Work out the finished part from the listing and answer in its coordinate system (mm). Round coordinates to 2 decimals unless told otherwise and drop trailing zeros. Order: outer loops, then holes, each group sorted by start corner. A loop starts at its lowest first (then second) coordinate and runs counter-clockwise, first axis right, second up. Notation, with made-up numbers: (21.25, 29.5) - (30.25, 29.5) arc R9 ccw to (30.25, 36.5) - close; hole circle Ø4 at (-22, -26.75). An arc over 180 degrees is marked (long way). Use one line per item in the form item = value. Start each with the question number.
Q1. The part is cut by section A-A on x = 328. Determine the outline of the cut face in (y, z), plus the area to 3 significant figures.
Q2. Find the intervals of material crossed by line 1 (X direction, y = 2.5, z = -352.5); line 2 (X direction, y = 6, z = 316); line 3 (Z direction, x = 98, y = 8.75), in increasing order. Write a range as [from, to].
Q3. The part is cut by section D-D on y = 8.5. State how many separate pieces and enclosed holes the cut face has, plus the area to 3 significant figures.
Q4. The part is cut by section C-C on x = -254.5. Determine the outline of the cut face in (y, z).
Q5. Given P1, Ø7, axis at x = -350, z = -322.5, coming from the -Y side; P2, Ø5, axis at y = 5.5, z = -165, coming from the -X side; P3, Ø5, axis at y = 6, z = -247, coming from the +X side, each flat-ended and moving along its own axis, determine where each tip first touches the part or whether it passes through.
Q6. The part is cut by section B-B on z = -23.5. Determine the outline of the cut face in (x, y), plus the area to 3 significant figures.
from build123d import *

# Parameters (mm, degrees)
SKETCH1_W           = 775
SKETCH1_H           = 735
BOSS_EXTRUDE1_DEPTH = 10
CUT_EXTRUDE1_DEPTH  = 10
SKETCH3_R           = 3.05
CUT_EXTRUDE2_DEPTH  = 10
CUT_EXTRUDE3_DEPTH  = 10
SKETCH5_R           = 4
CUT_EXTRUDE4_DEPTH  = 10
SKETCH6_R           = 3.05
CUT_EXTRUDE5_DEPTH  = 10
SKETCH7_R           = 8
CUT_EXTRUDE6_DEPTH  = 10


with BuildPart() as part:
    # Sketch1 → Boss-Extrude1 (new body)
    with BuildSketch(Plane(origin=(0, 0, 0), x_dir=(1, 0, 0), z_dir=(0, 1, 0))):
        Rectangle(SKETCH1_W, SKETCH1_H)
    extrude(amount=BOSS_EXTRUDE1_DEPTH)

    # Sketch2 → Cut-Extrude1 (cut)
    with BuildSketch(Plane(origin=(0, 10, 0), x_dir=(1, 0, 0), z_dir=(0, 1, 0))):
        Polygon((387.5, 307.5), (318.5, 307.5), (318.5, 79.5), (198.5, 79.5), (198.5, -0.5), (387.5, -0.5), align=None)
        Polygon((-387.5, -0.5), (-387.5, 307.5), (-318.5, 307.5), (-318.5, 79.5), (-198.5, 79.5), (-198.5, -0.5), align=None)
    extrude(amount=-CUT_EXTRUDE1_DEPTH, mode=Mode.SUBTRACT)

    # Sketch3 → Cut-Extrude2 (cut)
    with BuildSketch(Plane(origin=(0, 10, 0), x_dir=(1, 0, 0), z_dir=(0, 1, 0))):
        with Locations(Location((-350, 322.5, 0), (0, 0, 270))):
            Circle(SKETCH3_R)
        with Locations(Location((350, 322.5, 0), (0, 0, 90))):
            Circle(SKETCH3_R)
        with Locations(Location((350, -322.5, 0), (0, 0, 270))):
            Circle(SKETCH3_R)
        with Locations(Location((-350, -322.5, 0), (0, 0, 90))):
            Circle(SKETCH3_R)
        with Locations(Location((350, -50, 0), (0, 0, 90))):
            Circle(SKETCH3_R)
        with Locations(Location((-350, -50, 0), (0, 0, 270))):
            Circle(SKETCH3_R)
        with Locations(Location((-350, 352.5, 0), (0, 0, 270))):
            Circle(SKETCH3_R)
        with Locations(Location((350, 352.5, 0), (0, 0, 90))):
            Circle(SKETCH3_R)
    extrude(amount=-CUT_EXTRUDE2_DEPTH, mode=Mode.SUBTRACT)

    # Sketch4 → Cut-Extrude3 (cut)
    with BuildSketch(Plane(origin=(0, 10, 0), x_dir=(1, 0, 0), z_dir=(0, 1, 0))):
        with BuildLine():
            Line((-301.3, -214.3), (-301.3, -189.3))
            ThreePointArc((-301.3, -189.3), (-304.4, -186.2), (-307.5, -189.3))
            Line((-307.5, -189.3), (-307.5, -214.3))
            ThreePointArc((-307.5, -214.3), (-304.4, -217.4), (-301.3, -214.3))
        make_face()
        with BuildLine():
            Line((-223.8, -92.3), (-198.8, -92.3))
            ThreePointArc((-198.8, -92.3), (-195.7, -89.2), (-198.8, -86.1))
            Line((-198.8, -86.1), (-223.8, -86.1))
            ThreePointArc((-223.8, -86.1), (-226.9, -89.2), (-223.8, -92.3))
        make_face()
        with BuildLine():
            Line((-121.3, -189.3), (-121.3, -214.3))
            ThreePointArc((-121.3, -214.3), (-118.2, -217.4), (-115.1, -214.3))
            Line((-115.1, -214.3), (-115.1, -189.3))
            ThreePointArc((-115.1, -189.3), (-118.2, -186.2), (-121.3, -189.3))
        make_face()
        with BuildLine():
            Line((-198.8, -311.3), (-223.8, -311.3))
            ThreePointArc((-223.8, -311.3), (-226.9, -314.4), (-223.8, -317.5))
            Line((-223.8, -317.5), (-198.8, -317.5))
            ThreePointArc((-198.8, -317.5), (-195.7, -314.4), (-198.8, -311.3))
        make_face()
        with BuildLine():
            Line((198.8, -317.5), (223.8, -317.5))
            ThreePointArc((223.8, -317.5), (226.9, -314.4), (223.8, -311.3))
            Line((223.8, -311.3), (198.8, -311.3))
            ThreePointArc((198.8, -311.3), (195.7, -314.4), (198.8, -317.5))
        make_face()
        with BuildLine():
            Line((115.1, -189.3), (115.1, -214.3))
            ThreePointArc((115.1, -214.3), (118.2, -217.4), (121.3, -214.3))
            Line((121.3, -214.3), (121.3, -189.3))
            ThreePointArc((121.3, -189.3), (118.2, -186.2), (115.1, -189.3))
        make_face()
        with BuildLine():
            Line((223.8, -86.1), (198.8, -86.1))
            ThreePointArc((198.8, -86.1), (195.7, -89.2), (198.8, -92.3))
            Line((198.8, -92.3), (223.8, -92.3))
            ThreePointArc((223.8, -92.3), (226.9, -89.2), (223.8, -86.1))
        make_face()
        with BuildLine():
            Line((307.5, -214.3), (307.5, -189.3))
            ThreePointArc((307.5, -189.3), (304.4, -186.2), (301.3, -189.3))
            Line((301.3, -189.3), (301.3, -214.3))
            ThreePointArc((301.3, -214.3), (304.4, -217.4), (307.5, -214.3))
        make_face()
    extrude(amount=-CUT_EXTRUDE3_DEPTH, mode=Mode.SUBTRACT)

    # Sketch5 → Cut-Extrude4 (cut)
    with BuildSketch(Plane(origin=(0, 10, 0), x_dir=(1, 0, 0), z_dir=(0, 1, 0))):
        with Locations(Location((70.742847262, -307.5, 0), (0, 0, 270))):
            Circle(SKETCH5_R)
        with Locations(Location((-60.166013255, -290, 0), (0, 0, 270))):
            Circle(SKETCH5_R)
    extrude(amount=-CUT_EXTRUDE4_DEPTH, mode=Mode.SUBTRACT)

    # Sketch6 → Cut-Extrude5 (cut)
    with BuildSketch(Plane(origin=(0, 10, 0), x_dir=(1, 0, 0), z_dir=(0, 1, 0))):
        with Locations(Location((-100.729526925, -183.528276794, 0), (0, 0, 270))):
            Circle(SKETCH6_R)
        with Locations(Location((-80.603260731, -183.522806678, 0), (0, 0, 270))):
            Circle(SKETCH6_R)
        with Locations(Location((-100.762904784, -60.720718711, 0), (0, 0, 270))):
            Circle(SKETCH6_R)
        with Locations(Location((-80.636638589, -60.715248594, 0), (0, 0, 270))):
            Circle(SKETCH6_R)
        with Locations(Location((80.636638589, -60.715248594, 0), (0, 0, 90))):
            Circle(SKETCH6_R)
        with Locations(Location((100.762904784, -60.720718711, 0), (0, 0, 90))):
            Circle(SKETCH6_R)
        with Locations(Location((80.603260731, -183.522806678, 0), (0, 0, 90))):
            Circle(SKETCH6_R)
        with Locations(Location((100.729526925, -183.528276794, 0), (0, 0, 90))):
            Circle(SKETCH6_R)
        with Locations(Location((-309.45, -32.749027869, 0), (0, 0, 270))):
            Circle(SKETCH6_R)
        with Locations(Location((-295.213665555, -32.749027869, 0), (0, 0, 270))):
            Circle(SKETCH6_R)
        with Locations(Location((309.45, -32.749027869, 0), (0, 0, 90))):
            Circle(SKETCH6_R)
        with Locations(Location((295.213665555, -32.749027869, 0), (0, 0, 90))):
            Circle(SKETCH6_R)
        with BuildLine():
            Line((-312.5, -17.974833276), (-312.5, -0.5))
            ThreePointArc((-312.5, -0.5), (-309.45, 2.55), (-306.4, -0.5))
            Line((-306.4, -0.5), (-306.4, -17.974833276))
            ThreePointArc((-306.4, -17.974833276), (-309.45, -21.024833276), (-312.5, -17.974833276))
        make_face()
        with BuildLine():
            Line((312.5, -17.974833276), (312.5, -0.5))
            ThreePointArc((312.5, -0.5), (309.45, 2.55), (306.4, -0.5))
            Line((306.4, -0.5), (306.4, -17.974833276))
            ThreePointArc((306.4, -17.974833276), (309.45, -21.024833276), (312.5, -17.974833276))
        make_face()
    extrude(amount=-CUT_EXTRUDE5_DEPTH, mode=Mode.SUBTRACT)

    # Sketch7 → Cut-Extrude6 (cut)
    with BuildSketch(Plane(origin=(0, 10, 0), x_dir=(1, 0, 0), z_dir=(0, 1, 0))):
        with Locations(Location((-203.494386399, 241.114555962, 0), (0, 0, 270))):
            Circle(SKETCH7_R)
        with Locations(Location((203.494386399, 241.114555962, 0), (0, 0, 90))):
            Circle(SKETCH7_R)
        with BuildLine():
            Line((-12.5, -10.502549855), (12.5, -10.502549855))
            ThreePointArc((12.5, -10.502549855), (15.6, -13.602549855), (12.5, -16.702549855))
            Line((12.5, -16.702549855), (-12.5, -16.702549855))
            ThreePointArc((-12.5, -16.702549855), (-15.6, -13.602549855), (-12.5, -10.502549855))
        make_face()
        with BuildLine():
            Line((-12.5, 140.176827164), (12.5, 140.176827164))
            ThreePointArc((12.5, 140.176827164), (15.6, 137.076827164), (12.5, 133.976827164))
            Line((12.5, 133.976827164), (-12.5, 133.976827164))
            ThreePointArc((-12.5, 133.976827164), (-15.6, 137.076827164), (-12.5, 140.176827164))
        make_face()
        with BuildLine():
            Line((-24.016219384, 253.614555962), (-24.016219384, 228.614555962))
            ThreePointArc((-24.016219384, 228.614555962), (-27.116219384, 225.514555962), (-30.216219384, 228.614555962))
            Line((-30.216219384, 228.614555962), (-30.216219384, 253.614555962))
            ThreePointArc((-30.216219384, 253.614555962), (-27.116219384, 256.714555962), (-24.016219384, 253.614555962))
        make_face()
        with BuildLine():
            Line((-80.216219384, 253.614555962), (-80.216219384, 228.614555962))
            ThreePointArc((-80.216219384, 228.614555962), (-83.316219384, 225.514555962), (-86.416219384, 228.614555962))
            Line((-86.416219384, 228.614555962), (-86.416219384, 253.614555962))
            ThreePointArc((-86.416219384, 253.614555962), (-83.316219384, 256.714555962), (-80.216219384, 253.614555962))
        make_face()
        with BuildLine():
            Line((80.216219384, 253.614555962), (80.216219384, 228.614555962))
            ThreePointArc((80.216219384, 228.614555962), (83.316219384, 225.514555962), (86.416219384, 228.614555962))
            Line((86.416219384, 228.614555962), (86.416219384, 253.614555962))
            ThreePointArc((86.416219384, 253.614555962), (83.316219384, 256.714555962), (80.216219384, 253.614555962))
        make_face()
        with BuildLine():
            Line((24.016219384, 253.614555962), (24.016219384, 228.614555962))
            ThreePointArc((24.016219384, 228.614555962), (27.116219384, 225.514555962), (30.216219384, 228.614555962))
            Line((30.216219384, 228.614555962), (30.216219384, 253.614555962))
            ThreePointArc((30.216219384, 253.614555962), (27.116219384, 256.714555962), (24.016219384, 253.614555962))
        make_face()
    extrude(amount=-CUT_EXTRUDE6_DEPTH, mode=Mode.SUBTRACT)


solid = part.part
Found:
q1.outline = (0, -367.5) - (10, -367.5) - (10, -307.5) - (0, -307.5) - close; (0, 0.5) - (10, 0.5) - (10, 367.5) - (0, 367.5) - close
q1.area = 4,270 mm²
q2.line_1 = [-387.5, -353.05], [-346.95, 346.95], [353.05, 387.5]
q2.line_2 = [-387.5, -226.46], [-196.14, 196.14], [226.46, 387.5]
q2.line_3 = [-367.5, 59.43], [62.01, 182.17], [184.89, 367.5]
q3.separate_pieces = 1
q3.enclosed_holes = 38
q3.area = 504,000 mm²
q4.outline = (0, -367.5) - (10, -367.5) - (10, -79.5) - (0, -79.5) - close; (0, 0.5) - (10, 0.5) - (10, 367.5) - (0, 367.5) - close
q5.P1 = 0
q5.P2 = -318.5
q5.P3 = 318.5
q6.outline = (-198.5, 0) - (198.5, 0) - (198.5, 10) - (-198.5, 10) - close
q6.area = 3,970 mm²
